from build123d import *

# Parameters (mm, degrees)
SKETCH1_W           = 22.606
SKETCH1_H           = 48.006
SKETCH1_R           = 1.4
BOSS_EXTRUDE1_DEPTH = 6.35
SKETCH2_R           = 2
CUT_EXTRUDE1_DEPTH  = 23.606
SKETCH3_R           = 2.4
SKETCH3_R_2         = 1.4
BOSS_EXTRUDE2_DEPTH = 2
FILLET1_R           = 0.5


with BuildPart() as part:
    # Sketch1 → Boss-Extrude1 (new body)
    with BuildSketch(Plane(origin=(0, 0, 0), x_dir=(1, 0, 0), z_dir=(0, 1, 0))):
        with Locations((11.43, 24.13)):
            Rectangle(SKETCH1_W, SKETCH1_H)
        with Locations((3.6835, 35.20575)):
            Circle(SKETCH1_R, mode=Mode.SUBTRACT)
        with Locations((19.2073, 2.78275)):
            Circle(SKETCH1_R, mode=Mode.SUBTRACT)
    extrude(amount=BOSS_EXTRUDE1_DEPTH)

    # Sketch2 → Cut-Extrude1 (cut, through all)
    with BuildSketch(Plane.ZY.offset(-0.127)):
        with Locations((-26.67, 3.175)):
            Circle(SKETCH2_R)
        with Locations((-11.43, 3.175)):
            Circle(SKETCH2_R)
    extrude(amount=-CUT_EXTRUDE1_DEPTH, mode=Mode.SUBTRACT)

    # Sketch3 → Boss-Extrude2 (add)
    with BuildSketch(Plane(origin=(0, 6.35, 0), x_dir=(1, 0, 0), z_dir=(0, 1, 0))):
        with Locations((3.6835, 35.20575)):
            Circle(SKETCH3_R)
        with Locations((3.6835, 35.20575)):
            Circle(SKETCH3_R_2, mode=Mode.SUBTRACT)
        with Locations((19.2073, 2.78275)):
            Circle(SKETCH3_R)
        with Locations((19.2073, 2.78275)):
            Circle(SKETCH3_R_2, mode=Mode.SUBTRACT)
    extrude(amount=BOSS_EXTRUDE2_DEPTH)

    # Fillet1
    fillet1_edges = [part.edges().sort_by_distance(p)[0] for p in [
        (1.2835, 6.35, -35.20575),
        (16.8073, 6.35, -2.78275),
    ]]
    fillet(fillet1_edges, radius=FILLET1_R)


solid = part.part
Source: CAD feature listing. Evaluate the final solid. Frame: model axes, mm. A direction names the side the tool comes from. Round coordinates to 2 decimals unless told otherwise and drop trailing zeros. Loops run counter-clockwise (first coordinate to the right, second up) from the corner with the lowest first, then second, coordinate; pieces in that order, holes last. Notation, with made-up numbers: (55.25, 31.25) - (101.25, 31.25) arc R23 ccw to (101.25, 41.25) - close; hole circle Ø10 at (59.5, 38.5). An arc over 180 degrees is marked (long way). Write item = value, one per line. Start each with the question number.
Item 1: First-contact query: pin 1 Ø4 at (x, z) = (9, -6.5) entering from +Y; pin 2 Ø11.5 at (x, z) = (10.5, -30.5) entering from +Y. Flat tips, straight axial feed; report the tip coordinate or a pass-through.
Item 2: Material intervals for line 1 (Y direction, x = 14.5, z = -11.43) (3 decimals); line 2 (Z direction, x = 10, y = 4.5); line 3 (Z direction, x = 6.5, y = 5), sorted ascending.
Item 3: Mould query, pull axis X, two halves, no side actions, for faces 3 (the face through (20.5, 4.12, -2.25)), 4 (the face through (3.38, 4.12, -33.84)), 5 (the face through (5, 8.35, -34)), 6 (the face through (4.791, 7.589, -33.077)). Classes: released by +X, released by -X, zero draft, split by the parting line, or undercut.
Item 4: Section query A-A on z = -26.67. Output: boundary loops of the cut face in (x, y) (3 decimals).
Item 5: Section query B-B on x = 10.25. Output: boundary loops of the cut face in (y, z) (3 decimals), plus the area to 3 significant figures.
Item 6: Reachability of faces 1 (the face through (0.127, 3, -24)), 2 (the face through (18.69, 7.54, -0.44)) from +Z, -Z, +X, -X, +Y, -Y: full face, straight path, thin tool, end or side. Return the list, or none.
Results list:
q1.pin_1 = 6.35
q1.pin_2 = 6.51
q2.line_1 = 0 to 1.175, 5.175 to 6.35
q2.line_2 = -48.13 to -28.17, -25.17 to -12.93, -9.93 to -0.13
q2.line_3 = -48.13 to -27.49, -25.85 to -12.25, -10.61 to -0.13
q3.face_3 = undercut
q3.face_4 = undercut
q3.face_5 = zero draft
q3.face_6 = split by the parting line
q4.outline = (0.127, 0) - (22.733, 0) - (22.733, 1.175) - (0.127, 1.175) - close; (0.127, 5.175) - (22.733, 5.175) - (22.733, 6.35) - (0.127, 6.35) - close
q5.outline = (0, -48.133) - (6.35, -48.133) - (6.35, -0.127) - (0, -0.127) - close; hole circle Ø4 at (3.175, -26.67); hole circle Ø4 at (3.175, -11.43)
q5.area = 280 mm²
q6.face_1 = +Z, -Z, -X, +Y, -Y
q6.face_2 = +Y
